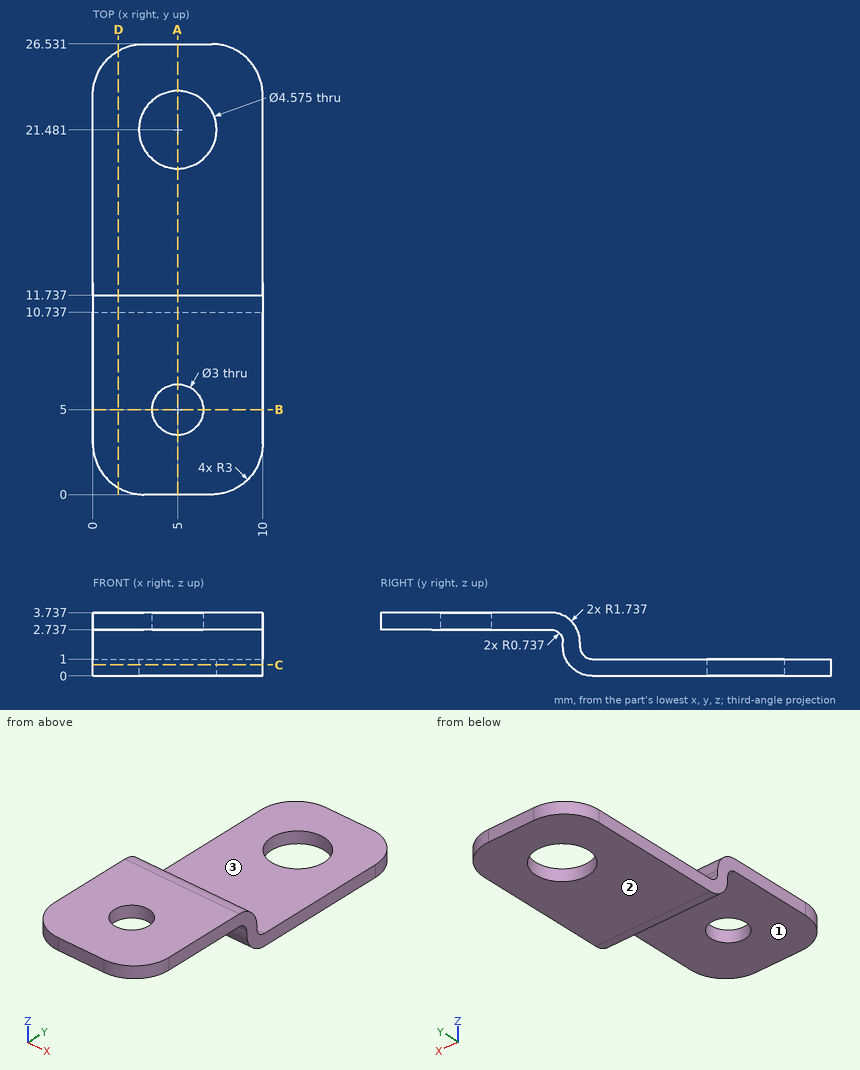
Source: three-view drawing plus pictorial views. Frame: mm from the lowest corner of the part. A direction names the side the tool comes from. Give positions to 0.01 mm unless a question says otherwise; leave off trailing zeros. Order: outer loops, then holes, each group sorted by start corner. A loop starts at its lowest first (then second) coordinate and runs counter-clockwise, first axis right, second up. Notation, with made-up numbers: M 77,-9.5 L 90,-9.5 A27 cw 90,13.5 Z; hole C 2.25,15 d3. An arc over 180 degrees is marked long. One line per question, with ' | ' between items. Start each with the question number.
1. Material intervals for probe 1 along Z at (x, y) = (1.5, 2.75); probe 2 along Y at (x, z) = (5, 2); probe 3 along Z at (x, y) = (0.75, 15), sorted ascending. Write a range as [from, to].
2. First-contact query: pin 1 Ø4 at (x, y) = (7.5, 19.5) entering from +Z; pin 2 Ø4 at (x, y) = (5, 5) entering from -Z. Flat tips, straight axial feed; report the tip coordinate or a pass-through.
3. Section query D-D (x = 1.5). Return the cut outline in (y, z).
4. Section query A-A (x = 5). Return the cut outline in (y, z).
5. Section query C-C (z = 0.65). Return the cut outline in (x, y) (1 decimal).
6. Section query B-B (y = 5). Return the cut outline in (x, z).
7. Access query for the marked faces 1, 2 and 3. Directions: +Z, -Z, +X, -X, +Y, -Y. A direction counts if a zero-diameter tool reaches every point of the face in a straight line with its end or side. Return the directions, or none.
Here are the results:
1) probe 1: [2.74, 3.74] | probe 2: [10.74, 11.74] | probe 3: [0, 1]
2) pin 1: z = 1 | pin 2: z = 2.74
3) outline: M 0.4,2.74 L 10,2.74 A0.74 cw 10.74,2 L 10.74,1.74 A1.74 ccw 12.47,0 L 26.13,0 L 26.13,1 L 12.47,1 A0.74 cw 11.74,1.74 L 11.74,2 A1.74 ccw 10,3.74 L 0.4,3.74 Z
4) outline: M 0,2.74 L 3.5,2.74 L 3.5,3.74 L 0,3.74 Z; M 6.5,2.74 L 10,2.74 A0.74 cw 10.74,2 L 10.74,1.74 A1.74 ccw 12.47,0 L 19.19,0 L 19.19,1 L 12.47,1 A0.74 cw 11.74,1.74 L 11.74,2 A1.74 ccw 10,3.74 L 6.5,3.74 Z; M 23.77,0 L 26.53,0 L 26.53,1 L 23.77,1 Z
5) outline: M 0,11.1 L 10,11.1 L 10,23.5 A3 ccw 7,26.5 L 3,26.5 A3 ccw 0,23.5 Z; hole C 5,21.5 d4.6
6) outline: M 0,2.74 L 3.5,2.74 L 3.5,3.74 L 0,3.74 Z; M 6.5,2.74 L 10,2.74 L 10,3.74 L 6.5,3.74 Z
7) face 1: -Z, +X, -X, -Y | face 2: -Z, +X, -X, +Y, -Y | face 3: +Z, +X, -X, +Y
